Can you work these out from the model? Positions are in its coordinate system, mm. Face numbers are marked on the shaded views. A direction names the side the tool comes from. Give positions to 0.01 mm unless a question says otherwise; leave off trailing zeros. Order: outer loops, then holes, each group sorted by start corner. A loop starts at its lowest first (then second) coordinate and runs counter-clockwise, first axis right, second up. Notation, with made-up numbers: (18.5, -22.75) - (69.5, -22.75) arc R8 cw to (69.5, -8.75) - close; hole circle Ø5 at (6.25, 60). An arc over 180 degrees is marked (long way). Return JSON: item names as keys, results as strings.
```python
from build123d import *

# Parameters (mm, degrees)
SKETCH1_R           = 50.8
SKETCH1_R_2         = 15.875
BOSS_EXTRUDE1_DEPTH = 9.525
SKETCH4_R           = 25.4
SKETCH4_R_2         = 15.875
BOSS_EXTRUDE2_DEPTH = 61.341
BOSS_EXTRUDE3_DEPTH = 4.7752
CIRPATTERN1_COUNT   = 4


with BuildPart() as part:
    # Sketch1 → Boss-Extrude1 (new body)
    with BuildSketch(Plane(origin=(0, 0, 0), x_dir=(1, 0, 0), z_dir=(0, 1, 0))):
        Circle(SKETCH1_R)
        Circle(SKETCH1_R_2, mode=Mode.SUBTRACT)
    extrude(amount=BOSS_EXTRUDE1_DEPTH)

    # Sketch4 → Boss-Extrude2 (add)
    with BuildSketch(Plane(origin=(0, 9.525, 0), x_dir=(1, 0, 0), z_dir=(0, 1, 0))):
        Circle(SKETCH4_R)
        Circle(SKETCH4_R_2, mode=Mode.SUBTRACT)
    extrude(amount=BOSS_EXTRUDE2_DEPTH)

    # Sketch7 → Boss-Extrude3 (add, symmetric)
    with BuildSketch(Plane.XY):
        Polygon((-25.4, 70.866), (-50.8, 9.525), (-22.583366139, 9.525), (-22.583366139, 70.866), align=None)
    boss_extrude3 = extrude(amount=BOSS_EXTRUDE3_DEPTH, both=True)

    # Sketch9 → 1/4 (0.375) Diameter Hole1 (revolve, cut)
    with BuildSketch(Plane(origin=(-26.940768363, 9.525, 26.940768363), x_dir=(0, 0, 1), z_dir=(1, 0, 0))):
        Polygon((0, 0), (0, 21.911598698), (4.7625, 19.05), (4.7625, 0), align=None)
    f_1_4_0_375_diameter_hole1 = revolve(axis=Axis((-26.940768363, 15.875, 26.940768363), (0, -1, 0)), mode=Mode.SUBTRACT)

    # CirPattern1: Boss-Extrude3, 1/4 (0.375) Diameter Hole1 ×4 about axis
    cirpattern1_axis = Axis((0, 0, 0), (0, 1, 0))
    for i in range(1, CIRPATTERN1_COUNT):
        add(boss_extrude3.rotate(cirpattern1_axis, i * 360 / CIRPATTERN1_COUNT))
        add(f_1_4_0_375_diameter_hole1.rotate(cirpattern1_axis, i * 360 / CIRPATTERN1_COUNT), mode=Mode.SUBTRACT)


solid = part.part
```
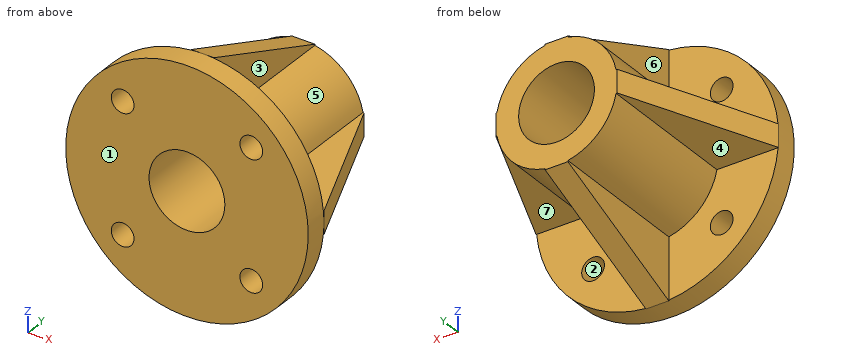
1. If I drill on L1, parallel to X at y = 18, z = 31; L2, parallel to Y at x = 23, z = -34 (3 decimals), over which ranges is the centre line in solid material (lowest first)? Write a range as [from, to].
Checks:
{"L1": "[-4.78, 4.78]", "L2": "[0, 9.525]"}
2. For pin 1 Ø8 at (y, z) = (16, 24.5) entering from +X; pin 2 Ø2 at (y, z) = (37.5, 2.5) entering from -X; pin 3 Ø1.5 at (x, z) = (39, 20.5) entering from +Y (3 decimals); pin 4 Ø15 at (x, z) = (-26.94, -26.94) entering from -Y, each with a flat end and sliding along its axis, tell me the tip position at first contact or that it passes through.
Checks:
{"pin 1": "x = 15", "pin 2": "x = -39.63", "pin 3": "y = 9.525", "pin 4": "y = 0"}
3. Suppose I cut it at B-B (y = 22.5). List the corners of the cut face in (x, z) for me (3 decimals).
Checks:
{"outline": "(-45.427, -4.775) - (-24.947, -4.775) arc R25.4 ccw to (-4.775, -24.947) - (-4.775, -45.427) - (4.775, -45.427) - (4.775, -24.947) arc R25.4 ccw to (24.947, -4.775) - (45.427, -4.775) - (45.427, 4.775) - (24.947, 4.775) arc R25.4 ccw to (4.775, 24.947) - (4.775, 45.427) - (-4.775, 45.427) - (-4.775, 24.947) arc R25.4 ccw to (-24.947, 4.775) - (-45.427, 4.775) - close; hole circle Ø31.75 at (0, 0)"}
4. Suppose I cut it at A-A (x = 11.5). List the corners of the cut face in (y, z) for me (3 decimals).
Checks:
{"outline": "(0, -49.481) - (9.525, -49.481) - (9.525, -22.648) - (70.866, -22.648) - (70.866, -10.944) - (0, -10.944) - close; (0, 10.944) - (70.866, 10.944) - (70.866, 22.648) - (9.525, 22.648) - (9.525, 49.481) - (0, 49.481) - close"}
5. Thinking about a two-plate mould opening in X: for the marked faces 1, 2 and 3, which applies, +X half, -X half, draft (parallel to the pull), parting line (faces both ways), or undercut?
Checks:
{"face 1": "draft", "face 2": "undercut", "face 3": "+X half"}
6. Suppose I cut it at C-C (z = 42). List the corners of the cut face in (x, y) for me (3 decimals), plus the area to 3 significant figures.
Checks:
{"outline": "(-28.577, 0) - (28.577, 0) - (28.577, 9.525) - (4.775, 9.525) - (4.775, 30.777) - (-4.775, 30.777) - (-4.775, 9.525) - (-28.577, 9.525) - close", "area": "747 mm^2"}
7. On a 3-axis mill with a long thin cutter (end or side, diameter ignored), from which of +Z, -Z, +X, -X, +Y, -Y can I reach the whole of each face in a straight line? I mean the marked faces 4, 5, 6 and 7. Say none if no direction works.
Checks:
{"face 4": "-Z, -X, +Y", "face 5": "+Z, +X, +Y", "face 6": "+Z, -X, +Y", "face 7": "-Z, +X, +Y"}
8. Suppose I cut it at D-D (x = 38). List the corners of the cut face in (y, z) for me (3 decimals).
Checks:
{"outline": "(0, -33.714) - (9.525, -33.714) - (9.525, -4.775) - (40.437, -4.775) - (40.437, 4.775) - (9.525, 4.775) - (9.525, 33.714) - (0, 33.714) - close"}
